Geometry check sheet. Reference: the model listing, model coordinates, mm. Face numbers are marked on the shaded views. Coordinates: 2 decimals unless noted, no trailing zeros. Loops run counter-clockwise (first coordinate to the right, second up) from the corner with the lowest first, then second, coordinate; pieces in that order, holes last. Notation, with made-up numbers: (-18, 61.5) - (-9, 61.5) arc R22 cw to (-9, 91.5) - close; hole circle Ø11 at (-13, 79). An arc over 180 degrees is marked (long way). Write each question's results on one line, items separated by ' | '. Start each with the question number.
(1) Material ranges on probe 1 along X at (y, z) = (-6.15, 15.5); probe 2 along X at (y, z) = (-3.25, -16); probe 3 along Y at (x, z) = (27, -15.35), recorded low to high.
(2) Mould release check, pull along Z, two halves, no side actions. Record for the marked faces 1, 2 and 3: pulls with the +Z half, pulls with the -Z half, needs draft (parallel to the pull), parting line crosses it, or undercut.
(3) Sectioned sample at A-A (z = 8). Enter the section's corners in (x, y), plus the area to 3 significant figures.
(4) Go/stop test with flat-tipped pins: pin 1 Ø1.5 at (y, z) = (-4, -12.5) entering from +X; pin 2 Ø4.5 at (x, z) = (-15.5, 15.5) entering from -Y; pin 3 Ø12 at (x, z) = (0, 0) entering from +Y. Record where each tip stops, or that it passes through.
(5) Sectioned sample at C-C (y = -1.25). Enter the section's corners in (x, z).
(6) Sectioned sample at B-B (x = -15.5). Enter the section's corners in (y, z).
(7) Sectioned sample at D-D (y = -6.5). Enter the section's corners in (x, z).
from build123d import *

# Parameters (mm, degrees)
F0_W           = 65
F0_H           = 36
F0_R           = 10
F1_DEPTH       = 8
F3_D           = 3.3
F3_CBORE_D     = 6.5
F3_CBORE_DEPTH = 3
F4_SIZE        = 0.5
F6_D           = 2.5
F6_DEPTH       = 13.5
F6_TIP         = 0.7510757738
F8_D           = 2.5
F8_DEPTH       = 13.5
F8_TIP         = 0.7510757738


with BuildPart() as f1:
    # F0 (on Front) → F1 (new body)
    with BuildSketch(Plane.XZ):
        Rectangle(F0_W, F0_H)
        Circle(F0_R, mode=Mode.SUBTRACT)
    extrude(amount=F1_DEPTH)

    # F3 (through all)
    with Locations(Plane.XZ.offset(8)):
        with Locations((15.5, 15.5), (-15.5, 15.5)):
            CounterBoreHole(F3_D / 2, F3_CBORE_D / 2, F3_CBORE_DEPTH)

    # F4
    f4_edges = [f1.edges().sort_by_distance(p)[0] for p in [
        (-32.5, -4, 18),
        (32.5, -4, 18),
        (32.5, -4, -18),
        (-32.5, -4, -18),
    ]]
    chamfer(f4_edges, length=F4_SIZE)

    # F6
    with Locations(Plane(origin=(0, 0, -18), x_dir=(1, 0, 0), z_dir=(0, 0, -1))):
        with Locations((27, 4), (-27, 4)):
            Hole(F6_D / 2, depth=F6_DEPTH)
            with Locations((0, 0, -(F6_DEPTH + F6_TIP / 2))):  # 118° drill point
                Cone(0, F6_D / 2, F6_TIP, mode=Mode.SUBTRACT)

    # F8
    with Locations(Plane.YZ.offset(32.5)):
        with Locations((-4, -12.5)):
            Hole(F8_D / 2, depth=F8_DEPTH)
            with Locations((0, 0, -(F8_DEPTH + F8_TIP / 2))):  # 118° drill point
                Cone(0, F8_D / 2, F8_TIP, mode=Mode.SUBTRACT)


solid = f1.part
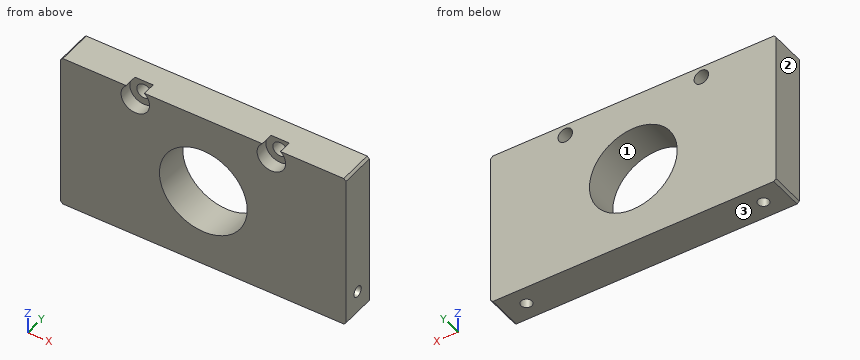
Outcome:
1) probe 1: x = -32.5 to -18.75, -12.25 to 12.25, 18.75 to 32.5 | probe 2: x = -32.5 to -28, -26 to 26, 28 to 32.5 | probe 3: y = -8 to -5.25, -2.75 to 0
2) face 1: undercut | face 2: needs draft | face 3: pulls with the -Z half
3) outline: (-32.5, -8) - (-6, -8) - (-6, 0) - (-32.5, 0) - close; (6, -8) - (32.5, -8) - (32.5, 0) - (6, 0) - close | area: 424 mm2
4) pin 1: stops at x = 18.7 | pin 2: stops at y = -5 | pin 3: passes through
5) outline: (-32.5, -17.5) - (-32, -18) - (32, -18) - (32.5, -17.5) - (32.5, 17.5) - (32, 18) - (-32, 18) - (-32.5, 17.5) - close; hole circle Ø3.3 at (-15.5, 15.5); hole circle Ø20 at (0, 0); hole circle Ø3.3 at (15.5, 15.5)
6) outline: (-8, -18) - (0, -18) - (0, 13.85) - (-5, 13.85) - (-5, 12.25) - (-8, 12.25) - close; (-5, 17.15) - (0, 17.15) - (0, 18) - (-5, 18) - close
7) outline: (-32.5, -17.5) - (-32, -18) - (32, -18) - (32.5, -17.5) - (32.5, 17.5) - (32, 18) - (17.58, 18) arc R3.25 cw (long way) to (13.42, 18) - (-13.42, 18) arc R3.25 cw (long way) to (-17.58, 18) - (-32, 18) - (-32.5, 17.5) - close; hole circle Ø20 at (0, 0)
